from build123d import *

# Parameters (mm, degrees)
BOSS_EXTRUDE1_DEPTH = 457.2
SKETCH2_W           = 50.8
SKETCH2_H           = 50.8
CUT_EXTRUDE1_DEPTH  = 22.225
CUT_EXTRUDE2_REACH  = 27.4
SKETCH3_R           = 2.667


with BuildPart() as part:
    # Sketch1 → Boss-Extrude1 (new body)
    with BuildSketch(Plane(origin=(0, 0, 0), x_dir=(0, 0, -1), z_dir=(1, 0, 0))):
        Polygon((3.175, 3.175), (3.175, 25.4), (0, 25.4), (0, 0), (50.8, 0), (50.8, 25.4), (47.625, 25.4), (47.625, 3.175), align=None)
    extrude(amount=BOSS_EXTRUDE1_DEPTH)

    # Sketch2 → Cut-Extrude1 (cut)
    with BuildSketch(Plane(origin=(0, 25.4, 0), x_dir=(1, 0, 0), z_dir=(0, 1, 0))):
        with Locations((25.4, 25.4)):
            Rectangle(SKETCH2_W, SKETCH2_H)
        with Locations((431.8, 25.4)):
            Rectangle(SKETCH2_W, SKETCH2_H)
    extrude(amount=-CUT_EXTRUDE1_DEPTH, mode=Mode.SUBTRACT)

    # Sketch3 → Cut-Extrude2 (cut, up to next)
    with BuildSketch(Plane.XZ, mode=Mode.PRIVATE) as cut_extrude2_sk1:
        with Locations((25.4, -25.4)):
            Circle(SKETCH3_R)
    cut_extrude2_tool1 = extrude(cut_extrude2_sk1.sketch, amount=-CUT_EXTRUDE2_REACH, mode=Mode.PRIVATE) & part.part
    add(cut_extrude2_tool1.solids().sort_by_distance((25.4, 0, -25.4))[0], mode=Mode.SUBTRACT)
    # Sketch3 → Cut-Extrude2 (cut, up to next)
    with BuildSketch(Plane.XZ, mode=Mode.PRIVATE) as cut_extrude2_sk2:
        with Locations((431.8, -25.4)):
            Circle(SKETCH3_R)
    cut_extrude2_tool2 = extrude(cut_extrude2_sk2.sketch, amount=-CUT_EXTRUDE2_REACH, mode=Mode.PRIVATE) & part.part
    add(cut_extrude2_tool2.solids().sort_by_distance((431.8, 0, -25.4))[0], mode=Mode.SUBTRACT)


solid = part.part
Build history of the part. All positions in model axes, mm. A direction names the side the tool comes from. Round coordinates to 2 decimals unless told otherwise and drop trailing zeros. Write each loop counter-clockwise with the first axis right and the second up, starting at its lowest first coordinate (ties: lowest second). Pieces come first, ordered by that corner, then holes. Notation, with made-up numbers: (-11, 60) - (41, 60) arc R34 ccw to (41, 93) - close; hole circle Ø11 at (89.25, 10). An arc over 180 degrees is marked (long way). Use CSV: the item, a comma, the result in double quotes.
(1) Wall check: line 1 (X direction, y = 2.75, z = -25.5); line 2 (Z direction, x = 77, y = 22.75) (3 decimals); line 3 (Z direction, x = 431.8, y = 1.65). Give the ranges that are in metal, low to high.
Response:
line 1,"0 to 22.73, 28.07 to 429.13, 434.47 to 457.2"
line 2,"-50.8 to -47.625, -3.175 to 0"
line 3,"-50.8 to -28.07, -22.73 to 0"
(2) Mould opens along Z. For faces 3 (the flat face through (225, 13, -50.8)), 4 (the flat face through (225, 0, -25)), 5 (the flat face through (226, 14, -3.175)) say: pulls with the +Z half, pulls with the -Z half, needs draft (parallel to the pull), parting line crosses it, or undercut.
Response:
face 3,"pulls with the -Z half"
face 4,"needs draft"
face 5,"undercut"
(3) 3-axis set-ups, long thin cutter, end or side, ignore diameter. For faces 1 (the flat face through (225, 13, 0)), 2 (the flat face through (226, 14, -47.625)): which of +Z, -Z, +X, -X, +Y, -Y reach the whole face in a straight line?
Response:
face 1,"+Z, +X, -X, +Y, -Y"
face 2,"+X, -X, +Y"
(4) Band-saw the part on C-C (z = -14). Write the cut outline in (x, y) (3 decimals).
Response:
outline,"(0, 0) - (457.2, 0) - (457.2, 3.175) - (0, 3.175) - close"
(5) Pin check, flat tips, straight feed: P1, Ø3, axis at x = 25.4, z = -25.4, coming from the +Y side; P2, Ø1.5, axis at x = 135, z = -18.5, coming from the +Y side (3 decimals); P3, Ø3.5, axis at y = 16, z = -1, coming from the +X side; P4, Ø1.6, axis at y = 13, z = -50, coming from the -X side. Stop position of each tip, or through.
Response:
P1,"through"
P2,"y = 3.175"
P3,"x = 406.4"
P4,"x = 50.8"
(6) Band-saw the part on B-B (x = 135). Write the cut outline in (y, z) (3 decimals), plus the area to 3 significant figures.
Response:
outline,"(0, -50.8) - (25.4, -50.8) - (25.4, -47.625) - (3.175, -47.625) - (3.175, -3.175) - (25.4, -3.175) - (25.4, 0) - (0, 0) - close"
area,"302 mm²"
(7) Band-saw the part on A-A (y = 7.5). Write the cut outline in (x, z) (3 decimals), plus the area to 3 significant figures.
Response:
outline,"(50.8, -50.8) - (406.4, -50.8) - (406.4, -47.625) - (50.8, -47.625) - close; (50.8, -3.175) - (406.4, -3.175) - (406.4, 0) - (50.8, 0) - close"
area,"2,260 mm²"
